Could you check a few things on this model? Use its own coordinates, in mm. A direction names the side the tool comes from. Round coordinates to 2 decimals unless told otherwise and drop trailing zeros. Write each loop counter-clockwise with the first axis right and the second up, starting at its lowest first coordinate (ties: lowest second). Pieces come first, ordered by that corner, then holes.
```python
from build123d import *

# Parameters (mm, degrees)
SKETCH1_W               = 39.624
SKETCH1_H               = 17.526
BOSS_EXTRUDE1_DEPTH     = 2.54
SKETCH2_R               = 1.517897845
CUT_EXTRUDE1_DEPTH      = 44.401309335
SKETCH3_R               = 6.35
BOSS_EXTRUDE2_DEPTH     = 15.24
SKETCH5_R               = 3.5052
CUT_EXTRUDE2_DEPTH      = 47.833219535
CUT_EXTRUDE3_REACH      = 45.438
CUT_EXTRUDE3_END_RADIUS = 3.5052
SKETCH6_R               = 1.1303
SKETCH7_R               = 2.38125
CUT_EXTRUDE4_DEPTH      = 1.27


with BuildPart() as part:
    # Sketch1 → Boss-Extrude1 (new body)
    with BuildSketch(Plane.XY):
        with Locations((19.812, -8.763)):
            Rectangle(SKETCH1_W, SKETCH1_H)
    extrude(amount=BOSS_EXTRUDE1_DEPTH)

    # Sketch2 → Cut-Extrude1 (cut, through all)
    with BuildSketch(Plane.XY.offset(2.54)):
        with Locations((36.83, -3.048)):
            Circle(SKETCH2_R)
        with Locations((21.5646, -14.478)):
            Circle(SKETCH2_R)
        with Locations((18.288, -3.048)):
            Circle(SKETCH2_R)
        with Locations((3.0226, -14.478)):
            Circle(SKETCH2_R)
    extrude(amount=-CUT_EXTRUDE1_DEPTH, mode=Mode.SUBTRACT)

    # Sketch3 → Boss-Extrude2 (add)
    with BuildSketch(Plane.XY.offset(2.54)):
        with Locations(Location((29.1973, -8.763, 0), (0, 0, 180))):
            Circle(SKETCH3_R)
    extrude(amount=BOSS_EXTRUDE2_DEPTH)

    # Sketch5 → Cut-Extrude2 (cut, through all)
    with BuildSketch(Plane.XY.offset(17.78)):
        with Locations((29.1973, -8.763)):
            Circle(SKETCH5_R)
    extrude(amount=-CUT_EXTRUDE2_DEPTH, mode=Mode.SUBTRACT)

    # Cut-Extrude3: up to this cylinder (the profile starts outside it)
    cut_extrude3_end = Plane(origin=(29.1973, -8.763, 11.43), z_dir=(0, 0, 1)) * Cylinder(CUT_EXTRUDE3_END_RADIUS, 98.8864, mode=Mode.PRIVATE)
    # Sketch6 → Cut-Extrude3 (cut, up to the surface)
    with BuildSketch(Plane(origin=(35.5473, 0, 0), x_dir=(0, 0, -1), z_dir=(1, 0, 0)), mode=Mode.PRIVATE) as cut_extrude3_sk1:
        with Locations((-11.43, -8.763)):
            Circle(SKETCH6_R)
    cut_extrude3_tool1 = extrude(cut_extrude3_sk1.sketch, amount=-CUT_EXTRUDE3_REACH, mode=Mode.PRIVATE) - cut_extrude3_end
    add(cut_extrude3_tool1.solids().sort_by_distance((35.5473, -8.763, 11.43))[0], mode=Mode.SUBTRACT)

    # Sketch7 → Cut-Extrude4 (cut)
    with BuildSketch(Plane(origin=(0, 0, 0), x_dir=(-1, 0, 0), z_dir=(0, 0, -1))):
        with Locations((-15.748, -14.224)):
            Circle(SKETCH7_R)
        with Locations((-5.715, -3.556)):
            Circle(SKETCH7_R)
        with Locations((-23.368, -3.556)):
            Circle(SKETCH7_R)
        with Locations((-33.274, -14.224)):
            Circle(SKETCH7_R)
    extrude(amount=-CUT_EXTRUDE4_DEPTH, mode=Mode.SUBTRACT)


solid = part.part
```
Q1. Imagine slicing it at B-B, the plane y = -10.5. Write out the boundary of the cut face in (x, z).
Q2. We'd pull the mould along X, two halves only. Please class faces 3 (the cylindrical face through (16.058, -11.863, 0.626)), 4 (the flat face through (15, -9, 2.54)), 5 (the cylindrical face through (23.14, -10.67, 10.05)): pulls with the +X half, pulls with the -X half, needs draft (parallel to the pull), parting line crosses it, or undercut.
Q3. Imagine slicing it at C-C, the plane z = 16. Write out the boundary of the cut face in (x, y).
Q4. Imagine slicing it at A-A, the plane x = 36.83. Write out the boundary of the cut face in (y, z).
Q5. On a 3-axis mill with a long thin cutter (end or side, diameter ignored), from which of +Z, -Z, +X, -X, +Y, -Y can I reach the whole of each face in a straight line? I mean faces 1 (the cylindrical face through (16.77, -2.98, 1.29)), 2 (the cylindrical face through (8.094, -3.451, 0.626)). Say none if no direction works.
Q6. I'm going to push flat-ended pins straight in: pin 1 Ø5 at (x, y) = (34, -15) entering from -Z; pin 2 Ø3.5 at (x, y) = (36.83, -3.048) entering from +Z; pin 3 Ø4 at (y, z) = (-10, 14) entering from -X; pin 4 Ø4.5 at (x, y) = (33.274, -14.224) entering from -Z. Where does each tip first touch, or does it pass through?
Q7. If I drill on L1, parallel to Y at x = 36.83, z = 1.5; L2, parallel to Z at x = 5.5, y = -5.5; L3, parallel to Z at x = 3.5, y = -12.75, over which ranges is the centre line in solid material (lowest first)?
Q8. Imagine slicing it at D-D, the plane x = 28.5. Write out the boundary of the cut face in (y, z), then the cut area to 3 significant figures.
Results found:
1. outline: (0, 0) - (26.15, 0) - (26.15, 17.78) - (23.09, 17.78) - (23.09, 2.54) - (0, 2.54) - close; (32.24, 0) - (39.62, 0) - (39.62, 2.54) - (35.31, 2.54) - (35.31, 17.78) - (32.24, 17.78) - close
2. face 3: undercut
2. face 4: needs draft
2. face 5: parting line crosses it
3. outline: circle Ø12.7 at (29.2, -8.76); hole circle Ø7.01 at (29.2, -8.76)
4. outline: (-17.53, 0) - (-4.57, 0) - (-4.57, 2.54) - (-17.53, 2.54) - close; (-1.53, 0) - (0, 0) - (0, 2.54) - (-1.53, 2.54) - close
5. face 1: +Z, -Z
5. face 2: -Z
6. pin 1: stops at z = 0
6. pin 2: stops at z = 2.54
6. pin 3: stops at x = 22.85
6. pin 4: stops at z = 1.27
7. L1: y = -17.53 to -4.57, -1.53 to 0
7. L2: z = 1.27 to 2.54
7. L3: z = 0 to 2.54
8. outline: (-17.53, 0) - (-12.2, 0) - (-12.2, 17.78) - (-15.07, 17.78) - (-15.07, 2.54) - (-17.53, 2.54) - close; (-5.33, 0) - (0, 0) - (0, 2.54) - (-2.45, 2.54) - (-2.45, 17.78) - (-5.33, 17.78) - close
8. area: 115 mm2
